from build123d import *

# Parameters (mm, degrees)
CONG_1_R                = 1.5
ESQUISSE3_R             = 0.9999999999999981
ESQUISSE3_R_2           = 1.0000000000000007
ENL_V_MAT_EXTRU_1_DEPTH = 62.583276982473095


with BuildPart() as part:
    # Balayage1: sweep along a path in Esquisse1
    with BuildLine(Plane(origin=(0, 0, 0), x_dir=(1, 0, 0), z_dir=(0, 1, 0))) as balayage1_path:
        Line((-33.5, 0), (-33.5, 11.999999999999943))
        ThreePointArc((-33.5, 11.999999999999943), (-31.156854249492383, 17.656854249492376), (-25.499999999999947, 20))
        Line((-25.499999999999947, 20), (25.499999999999947, 20))
        ThreePointArc((25.499999999999947, 20), (31.156854249492383, 17.65685424949238), (33.5, 11.999999999999943))
        Line((33.5, 11.999999999999943), (33.5, 0))
    # Esquisse2 → Balayage1 (sweep)
    with BuildSketch(Plane.XY):
        with BuildLine():
            Line((-33.5, 0), (-33.5, 20))
            ThreePointArc((-33.5, 20), (-34.804210711669924, 21.487167292060715), (-36.448888739433606, 20.388228567653773))
            Line((-36.448888739433606, 20.388228567653773), (-41.07810147691004, 3.111771432346228))
            ThreePointArc((-41.07810147691004, 3.111771432346228), (-41.613848072830564, 2.3099699895631494), (-42.52699021634365, 2))
            Line((-42.52699021634365, 2), (-47.5, 2))
            Line((-47.5, 2), (-47.5, 0))
            Line((-47.5, 0), (-33.5, 0))
        make_face()
    sweep(path=balayage1_path.line)

    # Congé1
    cong_1_edges = [part.edges().sort_by_distance(p)[0] for p in [
        (-47.5, 2, -5.999999999999972),
        (-41.056349186103986, 2, -27.556349186104107),
        (1.8119e-13, 2, -33.999999999999666),
        (41.05634918610424, 2, -27.556349186103848),
        (33.5, 10, 0),
        (34.80421071166993, 21.487167292060715, 4.086e-14),
        (38.7634951081718, 11.750000000000082, 1.4287e-13),
        (41.613848072830564, 2.3099699895631502, 2.4514e-13),
        (45.0134951081715, 2, 3.1274e-13),
        (47.5, 1, 3.8014e-13),
        (47.49999999999984, 2, -5.999999999999591),
        (-47.5, 1, 0),
        (-45.013495108171824, 2, 0),
        (-41.613848072830564, 2.3099699895631502, 0),
        (-38.763495108171824, 11.75, 0),
        (-34.80421071166993, 21.487167292060715, 0),
        (-33.5, 10, 0),
    ]]
    fillet(cong_1_edges, radius=CONG_1_R)

    # Esquisse3 → Enlèv. mat.-Extru.1 (cut, through all)
    with BuildSketch(Plane(origin=(0, 2, 0), x_dir=(1, 0, 0), z_dir=(0, 1, 0))):
        with Locations(Location((-44.5, 5, 0), (0, 0, 270))):
            Circle(ESQUISSE3_R)
        with Locations(Location((-18.5, 31.000000000000004, 0), (0, 0, 270))):
            Circle(ESQUISSE3_R_2)
        with Locations(Location((44.5, 5, 0), (0, 0, 90))):
            Circle(ESQUISSE3_R)
        with Locations(Location((18.5, 31.000000000000004, 0), (0, 0, 90))):
            Circle(ESQUISSE3_R_2)
    extrude(amount=-ENL_V_MAT_EXTRU_1_DEPTH, mode=Mode.SUBTRACT)


solid = part.part
Design review of the part built by this model. Coordinates are the model's own, in mm. A direction names the side the tool comes from. Round coordinates to 2 decimals unless told otherwise and drop trailing zeros. Loops run counter-clockwise (first coordinate to the right, second up) from the corner with the lowest first, then second, coordinate; pieces in that order, holes last. Notation, with made-up numbers: (21.5, 20.25) - (77.5, 20.25) arc R13 ccw to (77.5, 37.25) - close; hole circle Ø6 at (-11.5, 74.5). An arc over 180 degrees is marked (long way). One line per question, with ' | ' between items.
1. Clearance check with flat-ended pins moving along their axes: P1, Ø1.2, axis at x = -18.5, z = -31, coming from the -Y side; P2, Ø2.5, axis at x = 18.5, z = -31, coming from the -Y side; P3, Ø11.5, axis at y = 7.5, z = -5, coming from the +X side; P4, Ø8.5, axis at y = 9, z = -8.5, coming from the -X side. State where each tip first meets the part, or that it passes through.
Results are:
P1: passes through | P2: stops at y = 0 | P3: stops at x = 46.83 | P4: stops at x = -40.64
2. For faces 4 (the face through (33.5, 10, -7)), 5 (the face through (0.36, 21.49, -21.33)), 6 (the face through (0, 2, -30)), list the 3-axis set-ups (+Z, -Z, +X, -X, +Y, -Y) from which the entire face can be reached by the end or side of a thin tool; tool diameter is ignored.
Results are:
face 4: +Z, +Y, -Y | face 5: +Y | face 6: -Z, +Y
3. We need section A-A, the plane z = -11. State the section outline as (x, y) points.
Results are:
outline: (-47.5, 0) - (-33.5, 0) - (-33.5, 20) arc R1.5 ccw to (-36.45, 20.39) - (-41.08, 3.11) arc R1.5 cw to (-42.53, 2) - (-46, 2) arc R1.5 ccw to (-47.5, 0.5) - close; (33.5, 0) - (47.5, 0) - (47.5, 0.5) arc R1.5 ccw to (46, 2) - (42.53, 2) arc R1.5 cw to (41.08, 3.11) - (36.45, 20.39) arc R1.5 ccw to (33.5, 20) - close
4. We need section C-C, the plane x = 18.5. State the section outline as (y, z) points, and give its area (3 significant figures).
Results are:
outline: (0, -34) - (0.5, -34) arc R1.5 ccw to (2, -32.5) - (2, -32) - (0, -32) - close; (0, -30) - (2, -30) - (2, -29.03) arc R1.5 cw to (3.11, -27.58) - (20.39, -22.95) arc R1.5 ccw to (20, -20) - (0, -20) - close | area: 126 mm²
5. For L1, parallel to X at y = 0.55, z = -5; L2, parallel to X at y = 0.5, z = -31; L3, parallel to X at y = 0.95, z = -5, list the stretches that pass through material, from the lowest coordinate up. Write a range as [from, to].
Results are:
L1: x = [-47.5, -45.5], [-43.5, -33.5], [33.5, 43.5], [45.5, 47.5] | L2: x = [-36.59, -19.5], [-17.5, 17.5], [19.5, 36.59] | L3: x = [-47.43, -45.5], [-43.5, -33.5], [33.5, 43.5], [45.5, 47.43]
6. Draft analysis for pull direction X (two halves, no side actions). For faces 1 (the face through (31.094, 10.14, -17.719)), 2 (the face through (38.38, 11.52, -0.45)), 3 (the face through (-41.23, 0.25, -27.38)), state which applies: released by +X, released by -X, zero draft, split by the parting line, or undercut.
Results are:
face 1: undercut | face 2: released by +X | face 3: released by -X
7. We need section B-B, the plane z = -5. State the section outline as (x, y) points, and give its area (3 significant figures).
Results are:
outline: (-47.5, 0) - (-45.5, 0) - (-45.5, 2) - (-46, 2) arc R1.5 ccw to (-47.5, 0.5) - close; (-43.5, 0) - (-33.5, 0) - (-33.5, 20) arc R1.5 ccw to (-36.45, 20.39) - (-41.08, 3.11) arc R1.5 cw to (-42.53, 2) - (-43.5, 2) - close; (33.5, 0) - (43.5, 0) - (43.5, 2) - (42.53, 2) arc R1.5 cw to (41.08, 3.11) - (36.45, 20.39) arc R1.5 ccw to (33.5, 20) - close; (45.5, 0) - (47.5, 0) - (47.5, 0.5) arc R1.5 ccw to (46, 2) - (45.5, 2) - close | area: 251 mm²
8. We need section D-D, the plane x = 5. State the section outline as (y, z) points.
Results are:
outline: (0, -34) - (0.5, -34) arc R1.5 ccw to (2, -32.5) - (2, -29.03) arc R1.5 cw to (3.11, -27.58) - (20.39, -22.95) arc R1.5 ccw to (20, -20) - (0, -20) - close
